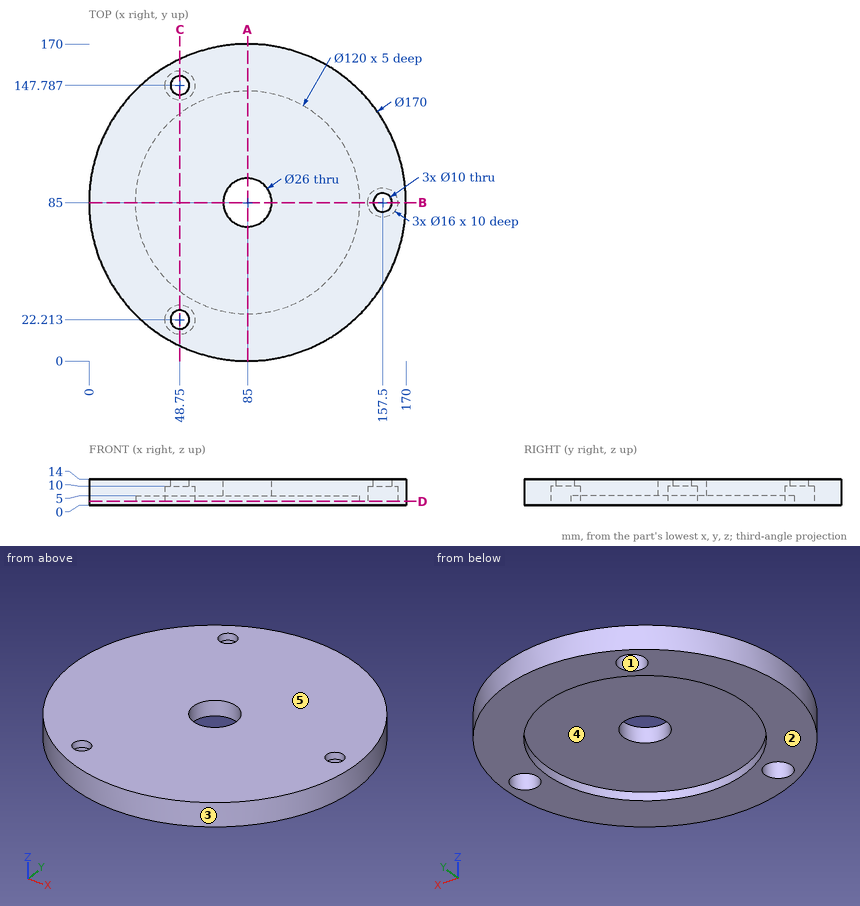
Design review of the part shown in the three views and the two pictorial views. Dimensions are in mm from the part's minimum x, y and z. A direction names the side the tool comes from. Round coordinates to 2 decimals unless told otherwise and drop trailing zeros. Loops run counter-clockwise (first coordinate to the right, second up) from the corner with the lowest first, then second, coordinate; pieces in that order, holes last. Notation, with made-up numbers: (30.25, 50) - (81.25, 50) arc R18 cw to (81.25, 71) - close; hole circle Ø8 at (-21, 30). An arc over 180 degrees is marked (long way). One line per item, written item: value. Start each with the question number.
Item 1: For the marked faces 4 and 5, list the 3-axis set-ups (+Z, -Z, +X, -X, +Y, -Y) from which the entire face can be reached by the end or side of a thin tool; tool diameter is ignored.
Item 2: Take a section at C-C (x = 48.75). Give the boundary of the cut face in (y, z).
Item 3: Clearance check with flat-ended pins moving along their axes: pin 1 Ø5 at (x, y) = (52, 149) entering from -Z; pin 2 Ø6 at (x, z) = (141, 10) entering from +Y; pin 3 Ø8 at (x, z) = (95.5, 11.5) entering from +Y. State where each tip first meets the part, or that it passes through.
Item 4: The part is to be moulded in two halves that separate along Y. For the marked faces 1, 2 and 3, say which applies: +Y half, -Y half, draft (parallel to the pull), parting line (faces both ways), or undercut.
Item 5: Take a section at D-D (z = 2). Give the boundary of the cut face in (x, y).
Item 6: Take a section at B-B (y = 85). Give the boundary of the cut face in (x, z).
Item 7: Take a section at A-A (x = 85). Give the boundary of the cut face in (y, z).
Item 8: For L1, parallel to Y at x = 48.75, z = 2.5; L2, parallel to Y at x = 85, z = 9; L3, parallel to Z at x = 61.5, y = 109.5, list the stretches that pass through material, from the lowest coordinate up.
Answer below:
1. face 4: -Z
1. face 5: +Z, +X, -X, +Y, -Y
2. outline: (8.12, 0) - (14.21, 0) - (14.21, 10) - (17.21, 10) - (17.21, 14) - (8.12, 14) - close; (27.21, 10) - (30.21, 10) - (30.21, 0) - (37.19, 0) - (37.19, 5) - (132.81, 5) - (132.81, 0) - (139.79, 0) - (139.79, 10) - (142.79, 10) - (142.79, 14) - (27.21, 14) - close; (152.79, 10) - (155.79, 10) - (155.79, 0) - (161.88, 0) - (161.88, 14) - (152.79, 14) - close
3. pin 1: stops at z = 10
3. pin 2: stops at y = 151.45
3. pin 3: stops at y = 169.75
4. face 1: undercut
4. face 2: draft
4. face 3: parting line
5. outline: circle Ø170 at (85, 85); hole circle Ø120 at (85, 85); hole circle Ø16 at (48.75, 22.21); hole circle Ø16 at (48.75, 147.79); hole circle Ø16 at (157.5, 85)
6. outline: (0, 0) - (25, 0) - (25, 5) - (72, 5) - (72, 14) - (0, 14) - close; (98, 5) - (145, 5) - (145, 0) - (149.5, 0) - (149.5, 10) - (152.5, 10) - (152.5, 14) - (98, 14) - close; (162.5, 10) - (165.5, 10) - (165.5, 0) - (170, 0) - (170, 14) - (162.5, 14) - close
7. outline: (0, 0) - (25, 0) - (25, 5) - (72, 5) - (72, 14) - (0, 14) - close; (98, 5) - (145, 5) - (145, 0) - (170, 0) - (170, 14) - (98, 14) - close
8. L1: y = 8.12 to 14.21, 30.21 to 37.19, 132.81 to 139.79, 155.79 to 161.88
8. L2: y = 0 to 72, 98 to 170
8. L3: z = 5 to 14
